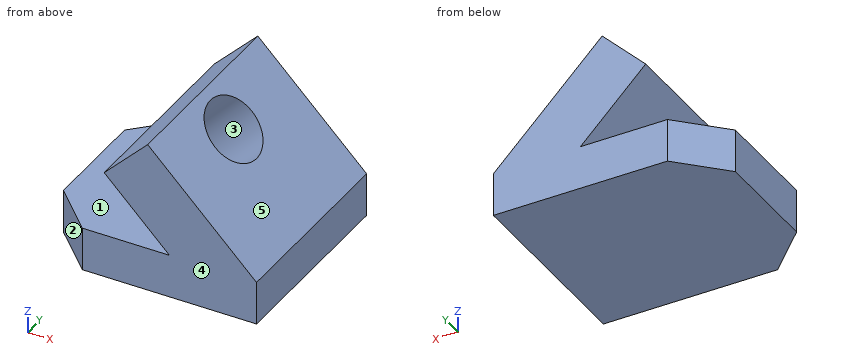
```python
from build123d import *

# Parameters (mm, degrees)
F1_DEPTH = 114.3
F3_DEPTH = 50.8
F5_DEPTH = 76.2


with BuildPart() as f1:
    # F0 (on Front) → F1 (new body, symmetric)
    with BuildSketch(Plane.XZ):
        Polygon((50.8, 50.8), (50.8, 0), (254, 0), (254, 50.8), (127, 177.8), (76.2, 127), (152.4, 50.8), align=None)
    extrude(amount=F1_DEPTH, both=True)

    # F2 (on face) → F3 (join)
    with BuildSketch(Plane(origin=(0, 0, 0), x_dir=(1, 0, 0), z_dir=(0, 0, -1))):
        Polygon((50.8, -114.3), (50.8, 114.3), (0, 63.5), (0, 0), (0, -63.5), align=None)
    extrude(amount=-F3_DEPTH)

    # F4 (on face) → F5 (cut, symmetric)
    with BuildSketch(Plane(origin=(152.4, 0, 152.4), x_dir=(0.707107, 0, -0.707107), z_dir=(0.707107, 0, 0.707107))):
        with BuildLine():
            ThreePointArc((52.978976, 0), (14.878976, 38.1), (-23.221024, 0))
            ThreePointArc((-23.221024, 0), (14.878976, -38.1), (52.978976, 0))
        make_face()
    extrude(amount=F5_DEPTH, both=True, mode=Mode.SUBTRACT)


solid = f1.part
```
Verification items for the finished model (mm, model axes). Face numbers are marked on the shaded views. A direction names the side the tool comes from. Coordinates: 2 decimals unless noted, no trailing zeros. Loops run counter-clockwise (first coordinate to the right, second up) from the corner with the lowest first, then second, coordinate; pieces in that order, holes last. Notation, with made-up numbers: (-4, 75) - (8, 75) arc R28 cw to (8, 95) - close; hole circle Ø3 at (-18.5, -16). An arc over 180 degrees is marked (long way). Put each result on its own line as item: value.
Item 1: Draft check along X on the marked faces 3, 4 and 5. Enter one of: pulls with the +X half, pulls with the -X half, needs draft (parallel to the pull), parting line crosses it, or undercut.
Conclusion:
face 3: undercut
face 4: needs draft
face 5: pulls with the +X half
Item 2: Gauge pin test, flat ends, axial feed: pin 1 Ø4 at (y, z) = (-91, 137) entering from -X; pin 2 Ø1 at (x, y) = (222, -81.5) entering from +Z; pin 3 Ø4 at (y, z) = (71, 58.5) entering from -X. Record the tip position at first contact, or that the pin passes through.
Conclusion:
pin 1: stops at x = 84.2
pin 2: stops at z = 83.3
pin 3: stops at x = 142.7
Item 3: Section check A-A (y = 68.5). Enter the section's corners in (x, z).
Conclusion:
outline: (5, 0) - (254, 0) - (254, 50.8) - (127, 177.8) - (76.2, 127) - (152.4, 50.8) - (5, 50.8) - close
Item 4: Scan lines: line 1 along Z through (x, y) = (128, -11); line 2 along Z through (x, y) = (137, 101.5); line 3 along Y through (x, z) = (20, 33). Record each from-to range of solid material in increasing order.
Conclusion:
line 1: z = 0 to 50.8, 158.54 to 176.8
line 2: z = 0 to 50.8, 66.2 to 167.8
line 3: y = -83.5 to 83.5
Item 5: Section check B-B (y = -23). Enter the section's corners in (x, z), then the cut area to 3 significant figures.
Conclusion:
outline: (0, 0) - (254, 0) - (254, 50.8) - (184.4, 120.4) - (133.6, 69.6) - (152.4, 50.8) - (0, 50.8) - close; (76.2, 127) - (90.64, 112.56) - (141.44, 163.36) - (127, 177.8) - close
area: 18,900 mm2
Item 6: Set-up check for the marked faces 1 and 2: record each of +Z, -Z, +X, -X, +Y, -Y from which the full face is reachable in a straight line by a thin tool's end or side.
Conclusion:
face 1: -X, +Y, -Y
face 2: +Z, -Z, -X, -Y
Item 7: Section check D-D (x = 44). Enter the section's corners in (y, z), then the cut area to 3 significant figures.
Conclusion:
outline: (-107.5, 0) - (107.5, 0) - (107.5, 50.8) - (-107.5, 50.8) - close
area: 10,900 mm2
Item 8: Section check C-C (z = 42). Enter the section's corners in (x, y), then the cut area to 3 significant figures.
Conclusion:
outline: (0, -63.5) - (50.8, -114.3) - (254, -114.3) - (254, 114.3) - (50.8, 114.3) - (0, 63.5) - close
area: 55,500 mm2
